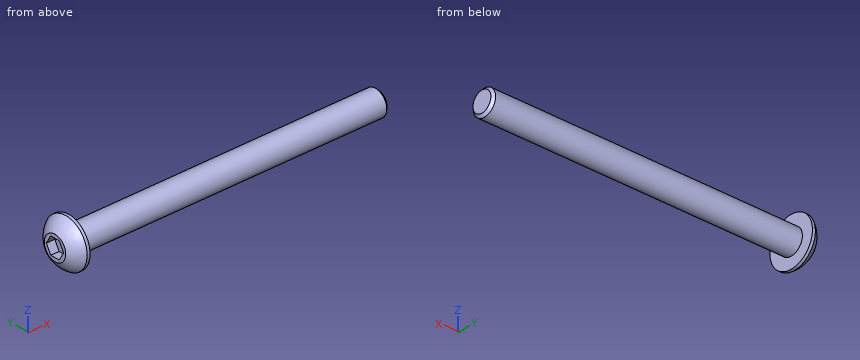
from build123d import *

# Parameters (mm, degrees)
CHAMFER1_SIZE      = 0.3
CUT_EXTRUDE1_DEPTH = 1


with BuildPart() as part:
    # Sketch1 → Revolve1 (revolve)
    with BuildSketch(Plane.XY, mode=Mode.PRIVATE) as revolve1_sk:
        with BuildLine():
            Line((0, 1.43), (0, 0))
            Line((0, 0), (38.65, 0))
            Line((38.65, 0), (38.65, 1.5))
            Line((38.65, 1.5), (1.65, 1.5))
            Line((1.65, 1.5), (1.65, 2.85))
            Line((1.65, 2.85), (1.3, 2.85))
            ThreePointArc((1.3, 2.85), (0.550445176, 2.231141741), (0, 1.43))
        make_face()
    revolve(revolve1_sk.sketch.rotate(Axis((0, 0, 0), (1, 0, 0)), 90), axis=Axis((0, 0, 0), (1, 0, 0)))

    # Chamfer1
    chamfer1_edges = [part.edges().sort_by_distance(p)[0] for p in [
        (38.65, 0, -1.5),
    ]]
    chamfer(chamfer1_edges, length=CHAMFER1_SIZE)

    # Sketch2 → Cut-Extrude1 (cut)
    with BuildSketch(Plane.ZY):
        Polygon((0, 1.154700538), (-1, 0.577350269), (-1, -0.577350269), (0, -1.154700538), (1, -0.577350269), (1, 0.577350269), align=None)
    extrude(amount=-CUT_EXTRUDE1_DEPTH, mode=Mode.SUBTRACT)


solid = part.part
Geometry check sheet. Reference: the model listing, model coordinates, mm. Coordinates: 2 decimals unless noted, no trailing zeros. Order: outer loops, then holes, each group sorted by start corner. A loop starts at its lowest first (then second) coordinate and runs counter-clockwise, first axis right, second up. Notation, with made-up numbers: (-8.75, 47.5) -> (46.25, 47.5) arc R36 ccw to (46.25, 83.5) -> close; hole circle Ø3 at (37.5, 22.5). An arc over 180 degrees is marked (long way). Use a Markdown table: item, result. Add a question column.
1. Go/stop test with flat-tipped pins: pin 1 Ø2 at (x, z) = (32, -1.5) entering from +Y; pin 2 Ø0.5 at (x, y) = (0.5, 0) entering from -Z; pin 3 Ø1.1 at (x, y) = (0.5, 0) entering from +Z. Record where each tip stops, or that it passes through.
2. Cross-section at A-A (x = 8). Enter the section's corners in (y, z).
3. Material ranges on L1, parallel to Z at x = 9.5, y = 0.45; L2, parallel to X at y = -0.85, z = -0.4, recorded low to high.
Filled sheet:
| question | item | result |
|---|---|---|
| 1 | pin 1 | y = 1.41 |
| 1 | pin 2 | z = -2.43 |
| 1 | pin 3 | z = 2.68 |
| 2 | outline | circle Ø3 at (0, 0) |
| 3 | L1 | -1.43 to 1.43 |
| 3 | L2 | 1 to 38.65 |
